```python
from build123d import *

# Parameters (mm, degrees)
SKETCH1_R           = 2.54
SKETCH1_R_2         = 1.797730585
BOSS_EXTRUDE1_DEPTH = 6.35
CUT_EXTRUDE1_DEPTH  = 90.090296329
FILLET1_R           = 6.35


with BuildPart() as part:
    # Sketch1 → Boss-Extrude1 (new body)
    with BuildSketch(Plane.XY):
        Polygon((21.59, 0), (76.2, 20.32), (76.2, 45.72), (0, 45.72), (0, 0), align=None)
        with Locations((10.795, 12.7)):
            Circle(SKETCH1_R, mode=Mode.SUBTRACT)
        with Locations((69.85, 39.37)):
            Circle(SKETCH1_R_2, mode=Mode.SUBTRACT)
        with Locations((57.15, 39.37)):
            Circle(SKETCH1_R_2, mode=Mode.SUBTRACT)
        with Locations((44.45, 39.37)):
            Circle(SKETCH1_R_2, mode=Mode.SUBTRACT)
        with Locations((31.75, 39.37)):
            Circle(SKETCH1_R_2, mode=Mode.SUBTRACT)
        with Locations((19.05, 39.37)):
            Circle(SKETCH1_R_2, mode=Mode.SUBTRACT)
        with Locations((6.35, 39.37)):
            Circle(SKETCH1_R_2, mode=Mode.SUBTRACT)
        with Locations((57.15, 26.67)):
            Circle(SKETCH1_R_2, mode=Mode.SUBTRACT)
        with Locations((44.45, 26.67)):
            Circle(SKETCH1_R_2, mode=Mode.SUBTRACT)
        with Locations((31.75, 26.67)):
            Circle(SKETCH1_R_2, mode=Mode.SUBTRACT)
        with Locations((19.05, 26.67)):
            Circle(SKETCH1_R_2, mode=Mode.SUBTRACT)
        with Locations((6.35, 26.67)):
            Circle(SKETCH1_R_2, mode=Mode.SUBTRACT)
        with Locations((69.85, 26.67)):
            Circle(SKETCH1_R_2, mode=Mode.SUBTRACT)
    extrude(amount=BOSS_EXTRUDE1_DEPTH)

    # Sketch2 → Cut-Extrude1 (cut, through all)
    with BuildSketch(Plane.XY.offset(6.35)):
        Polygon((17.78, 0), (17.78, 2.54), (27.186735348, 19.105501202), (45.29738426, 8.821352283), (21.59, 0), align=None)
    extrude(amount=-CUT_EXTRUDE1_DEPTH, mode=Mode.SUBTRACT)

    # Fillet1
    # the kernel refuses this fillet: 6.35 mm, written as the material it adds along each edge
    with BuildSketch(Plane(origin=(27.186735348, 19.105501202, 6.35), x_dir=(0.8695801156095444, -0.4937918818049677, 0), z_dir=(0, 0, -1))) as fillet1_piece_1:
        with BuildLine():
            CenterArc((FILLET1_R, FILLET1_R), FILLET1_R, 180, 90)
            Line((0, FILLET1_R), (0, 0))
            Line((0, 0), (FILLET1_R, 0))
        make_face()
    extrude(amount=6.35)
    # the kernel refuses this fillet: 6.35 mm, written as the material it takes off along each edge
    with BuildSketch(Plane(origin=(45.29738426, 8.821352283, 13.752634073), x_dir=(0.9372218510575621, 0.3487337120214175, 0), z_dir=(0, 0, -1))) as fillet1_2_piece_1:
        with BuildLine():
            CenterArc((FILLET1_R * 0.466307658155, -FILLET1_R), FILLET1_R, 90, 50)
            Line((-FILLET1_R * 0.299736784964, -FILLET1_R * 0.357212390313), (0, 0))
            Line((0, 0), (FILLET1_R * 0.466307658155, 0))
        make_face()
    extrude(amount=21.155268146, mode=Mode.SUBTRACT)
    with BuildSketch(Plane(origin=(76.2, 20.32, -11.031382068), x_dir=(-0.9372218510575616, -0.34873371202141845, 0), z_dir=(0, 0, 1))) as fillet1_2_piece_2:
        with BuildLine():
            CenterArc((FILLET1_R * 0.694890209019, -FILLET1_R), FILLET1_R, 90, 69.590117166)
            Line((-FILLET1_R * 0.242331642039, -FILLET1_R * 0.651266287979), (0, 0))
            Line((0, 0), (FILLET1_R * 0.694890209019, 0))
        make_face()
    extrude(amount=28.412764136, mode=Mode.SUBTRACT)
    with BuildSketch(Plane(origin=(76.2, 45.72, -15.875), x_dir=(0, -1, 0), z_dir=(0, 0, 1))) as fillet1_2_piece_3:
        with BuildLine():
            CenterArc((FILLET1_R, -FILLET1_R), FILLET1_R, 90, 90)
            Line((0, -FILLET1_R), (0, 0))
            Line((0, 0), (FILLET1_R, 0))
        make_face()
    extrude(amount=38.1, mode=Mode.SUBTRACT)
    with BuildSketch(Plane(origin=(0, 45.72, -15.875), x_dir=(0, -1, 0), z_dir=(0, 0, 1)), Plane(origin=(0, 0, -15.875), x_dir=(1, 0, 0), z_dir=(0, 0, 1))) as fillet1_2_piece_4:
        with BuildLine():
            CenterArc((FILLET1_R, FILLET1_R), FILLET1_R, 180, 90)
            Line((0, FILLET1_R), (0, 0))
            Line((0, 0), (FILLET1_R, 0))
        make_face()
    extrude(amount=38.1, mode=Mode.SUBTRACT)
    with BuildSketch(Plane(origin=(17.78, 0, 19.05), x_dir=(0, 1, 0), z_dir=(0, 0, -1))) as fillet1_2_piece_5:
        with BuildLine():
            CenterArc((6.35, -5.08), FILLET1_R, 126.869897646, 53.130102354)
            Line((0, -5.08), (0, 0))
            Line((0, 0), (2.54, 0))
        make_face()
    extrude(amount=31.75, mode=Mode.SUBTRACT)


solid = part.part
```
Work out the finished part from the listing and answer in its coordinate system (mm). A direction names the side the tool comes from. Give positions to 0.01 mm unless a question says otherwise; leave off trailing zeros. Write each loop counter-clockwise with the first axis right and the second up, starting at its lowest first coordinate (ties: lowest second). Pieces come first, ordered by that corner, then holes. Notation, with made-up numbers: (5, 16.25) -> (40, 16.25) arc R37 cw to (40, 54.25) -> close; hole circle Ø11 at (86, 11). An arc over 180 degrees is marked (long way). Write each question's results on one line, items separated by ' | '.
1. Find section D-D on x = 50.5. Determine the outline of the cut face in (y, z), and give its area (3 significant figures).
Data:
outline: (10.76, 0) -> (45.72, 0) -> (45.72, 6.35) -> (10.76, 6.35) -> close | area: 222 mm^2
2. Determine the mould class of faces 1 (the cylindrical face through (44.06, 37.615, 3.131)), 2 (the cylindrical face through (15.6, 0.7, 3.2)), 3 (the cylindrical face through (1.9, 43.9, 3.1)), 4 (the flat face through (76.2, 32, 3)) for opening direction Y: +Y half, -Y half, draft (parallel to the pull), parting line (faces both ways), or undercut.
Data:
face 1: undercut | face 2: -Y half | face 3: +Y half | face 4: draft
3. Straight lines are drawn through the part: L1, parallel to Y at x = 44.45, z = 5; L2, parallel to Y at x = 6, z = 6; L3, parallel to Y at x = 11, z = 3.25. For each, find the intervals that lie inside material, in ascending order.
Data:
L1: 9.61 to 24.87, 28.47 to 37.57, 41.17 to 45.72 | L2: 0.01 to 24.91, 28.43 to 37.61, 41.13 to 45.71 | L3: 0 to 10.17, 15.23 to 45.72
4. Find section B-B on y = 12.7. Determine the outline of the cut face in (x, z) (3 decimals), and give its area (3 significant figures).
Data:
outline: (0, 0) -> (8.255, 0) -> (8.255, 6.35) -> (0, 6.35) -> close; (13.335, 0) -> (23.549, 0) -> (23.549, 6.35) -> (13.335, 6.35) -> close; (38.467, 0) -> (55.721, 0) -> (55.721, 6.35) -> (38.467, 6.35) -> close | area: 227 mm^2
5. A tool of negligible diameter and unlimited length cuts with its end or side. For faces 5 (the cylindrical face through (32.58, 37.775, 3.131)), 6 (the flat face through (20.87, 7.98, 3.22)), from which of +Z, -Z, +X, -X, +Y, -Y can it reach the whole face along a straight path? Write none if from no direction.
Data:
face 5: +Z, -Z | face 6: +Z, -Z, -Y
6. Find section C-C on z = 5. Give the number of separate pieces and of enclosed holes in the cut face, and give its area (3 significant figures).
Data:
separate pieces: 1 | enclosed holes: 13 | area: 2,510 mm^2
7. Find section A-A on x = 20. Determine the outline of the cut face in (y, z), and give its area (3 significant figures).
Data:
outline: (6.45, 0) -> (25.14, 0) -> (25.14, 6.35) -> (6.45, 6.35) -> close; (28.2, 0) -> (37.84, 0) -> (37.84, 6.35) -> (28.2, 6.35) -> close; (40.9, 0) -> (45.72, 0) -> (45.72, 6.35) -> (40.9, 6.35) -> close | area: 211 mm^2
8. Each of these flat-tipped pins is pushed along its axis until it touches: pin 1 Ø1.5 at (y, z) = (21.5, 1) entering from +X; pin 2 Ø4 at (x, y) = (7.5, 14) entering from -Z; pin 3 Ø3 at (y, z) = (20, 4) entering from +X. Where does it stop, or does it pass through?
Data:
pin 1: x = 75.69 | pin 2: z = 0 | pin 3: x = 75.32
